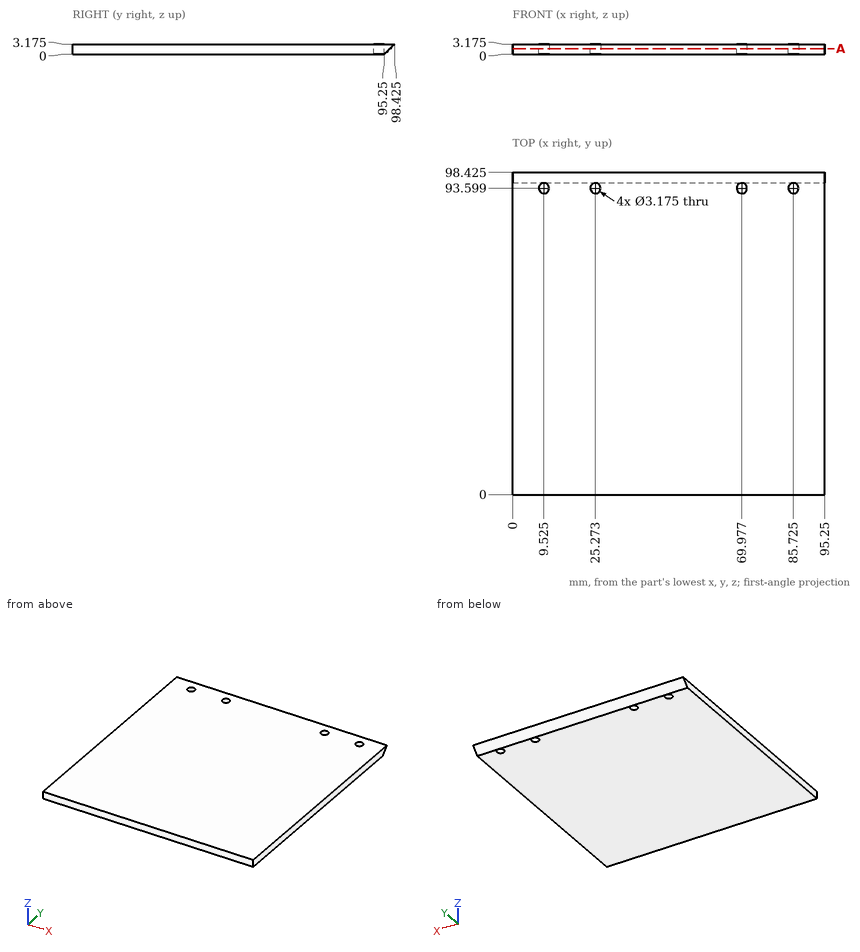
For this review, use the dimensioned drawing (mm, ordinates from the lowest corner) and the shaded views. Coordinates: 2 decimals unless noted, no trailing zeros. Use a Markdown table: item, result. Add a question column.
1. To check wall thickness, follow line 1 (Y direction, x = 26, z = 0.2); line 2 (Y direction, x = 48, z = 0.25); line 3 (Y direction, x = 4.5, z = 2.25). State the ranges of each line that lie inside material, in increasing order.
2. Add section A-A on z = 1.75. Give the number of separate pieces and of enclosed holes in the cut face, plus the area to 3 significant figures.
3. Clearance check with a flat-ended pin moving along its axis: pin 1 Ø1.9 at (x, y) = (9.525, 93.599) entering from +Z. State where the tip first meets the part, or that it passes through.
Returned:
| question | item | result |
|---|---|---|
| 1 | line 1 | y = 0 to 92.19, 95.01 to 95.45 |
| 1 | line 2 | y = 0 to 95.5 |
| 1 | line 3 | y = 0 to 97.5 |
| 2 | separate pieces | 1 |
| 2 | enclosed holes | 4 |
| 2 | area | 9,210 mm² |
| 3 | pin 1 | passes through |
